from build123d import *

# Parameters (mm, degrees)
SKETCH1_R           = 19.05
BOSS_EXTRUDE1_DEPTH = 3.175
SKETCH2_R           = 12.065
CUT_EXTRUDE1_DEPTH  = 28.127211891
SKETCH3_R           = 13.335
CUT_EXTRUDE2_DEPTH  = 1.5875
BOSS_EXTRUDE2_START = 15.24
SKETCH4_W           = 6.35
SKETCH4_H           = 6.35
BOSS_EXTRUDE2_DEPTH = 9.525
FILLET1_R           = 2.54
SKETCH5_R           = 1.7272
CUT_EXTRUDE3_DEPTH  = 7.62
FILLET2_R           = 1.3208
FILLET3_R           = 0.127
SKETCH6_R           = 1.1303
CUT_EXTRUDE4_DEPTH  = 32.405228218


with BuildPart() as part:
    # Sketch1 → Boss-Extrude1 (new body)
    with BuildSketch(Plane.XY):
        Circle(SKETCH1_R)
    extrude(amount=BOSS_EXTRUDE1_DEPTH)

    # Sketch2 → Cut-Extrude1 (cut, through all)
    with BuildSketch(Plane.XY.offset(3.175)):
        Circle(SKETCH2_R)
    extrude(amount=-CUT_EXTRUDE1_DEPTH, mode=Mode.SUBTRACT)

    # Sketch3 → Cut-Extrude2 (cut)
    with BuildSketch(Plane.XY.offset(3.175)):
        Circle(SKETCH3_R)
    extrude(amount=-CUT_EXTRUDE2_DEPTH, mode=Mode.SUBTRACT)

    # Sketch4 → Boss-Extrude2 (add)
    with BuildSketch(Plane(origin=(0, 0, 0), x_dir=(0, 0, -1), z_dir=(1, 0, 0)).offset(BOSS_EXTRUDE2_START)):
        with Locations((-3.175, 0)):
            Rectangle(SKETCH4_W, SKETCH4_H)
    extrude(amount=BOSS_EXTRUDE2_DEPTH)

    # Fillet1
    fillet1_edges = [part.edges().sort_by_distance(p)[0] for p in [
        (18.783553311, -3.175, 1.5875),
        (18.783553311, 3.175, 1.5875),
    ]]
    fillet(fillet1_edges, radius=FILLET1_R)

    # Sketch5 → Cut-Extrude3 (cut)
    with BuildSketch(Plane(origin=(24.765, 0, 0), x_dir=(0, 0, -1), z_dir=(1, 0, 0))):
        with Locations((-3.175, 0)):
            Circle(SKETCH5_R)
    extrude(amount=-CUT_EXTRUDE3_DEPTH, mode=Mode.SUBTRACT)

    # Fillet2
    fillet2_edges = [part.edges().sort_by_distance(p)[0] for p in [
        (15.24, 0, 3.175),
        (15.24, 0, 6.35),
    ]]
    fillet(fillet2_edges, radius=FILLET2_R)

    # Fillet3
    # the kernel refuses this fillet: 0.127 mm, written as the material it takes off along each edge
    with BuildSketch(Plane(origin=(0, 0, 3.175), x_dir=(1, 0, 0), z_dir=(0, -1, 0))) as fillet3_piece_1:
        with BuildLine():
            CenterArc((13.335 + FILLET3_R, -FILLET3_R), FILLET3_R, 90, 90)
            Line((13.335, -FILLET3_R), (13.335, 0))
            Line((13.335, 0), (13.335 + FILLET3_R, 0))
        make_face()
    revolve(axis=Axis((0, 0, 3.175), (0, 0, 1)), mode=Mode.SUBTRACT)
    with BuildSketch(Plane(origin=(0, 0, 1.5875), x_dir=(1, 0, 0), z_dir=(0, -1, 0))) as fillet3_piece_2:
        with BuildLine():
            CenterArc((12.065 + FILLET3_R, -FILLET3_R), FILLET3_R, 90, 90)
            Line((12.065, -FILLET3_R), (12.065, 0))
            Line((12.065, 0), (12.065 + FILLET3_R, 0))
        make_face()
    revolve(axis=Axis((0, 0, 1.5875), (0, 0, 1)), mode=Mode.SUBTRACT)
    with BuildSketch(Plane(origin=(16.5608, -3.175, 6.35), x_dir=(0, 0, -1), z_dir=(1, 0, 0))) as fillet3_piece_3:
        with BuildLine():
            CenterArc((FILLET3_R, FILLET3_R), FILLET3_R, 180, 90)
            Line((0, FILLET3_R), (0, 0))
            Line((0, 0), (FILLET3_R, 0))
        make_face()
    extrude(amount=8.5217, mode=Mode.SUBTRACT)
    with BuildSketch(Plane(origin=(16.5608, 3.175, 6.35), x_dir=(0, 0, -1), z_dir=(1, 0, 0))) as fillet3_piece_4:
        with BuildLine():
            CenterArc((FILLET3_R, -FILLET3_R), FILLET3_R, 90, 90)
            Line((0, -FILLET3_R), (0, 0))
            Line((0, 0), (FILLET3_R, 0))
        make_face()
    extrude(amount=8.5217, mode=Mode.SUBTRACT)
    with BuildSketch(Plane(origin=(0, 0, 3.175), x_dir=(0.9643291947502942, 0.2647058823529412, 0), z_dir=(0.2647058823529412, -0.9643291947502942, 0))) as fillet3_piece_5:
        with BuildLine():
            CenterArc((19.05 - FILLET3_R, -FILLET3_R), FILLET3_R, 0, 90)
            Line((19.05 - FILLET3_R, 0), (19.05, 0))
            Line((19.05, 0), (19.05, -FILLET3_R))
        make_face()
    revolve(axis=Axis((0, 0, 3.175), (0, 0, 1)), revolution_arc=329.301045966, mode=Mode.SUBTRACT)
    with BuildSketch(Plane(origin=(20.819867315, 5.715, 3.175), x_dir=(0.12470900704731759, -0.9921933599663284, 0), z_dir=(0.9921933599663284, 0.12470900704731759, 0))) as fillet3_piece_6_section:
        with BuildLine():
            CenterArc((2.54 + FILLET3_R, FILLET3_R), FILLET3_R, 180, 90)
            Line((2.54, FILLET3_R), (2.54, 0))
            Line((2.54, 0), (2.54 + FILLET3_R, 0))
        make_face()
    fillet3_piece_6 = revolve(axis=Axis((20.819867315, 5.715, 3.175), (0, 0, -1)), revolution_arc=81.814474605, mode=Mode.PRIVATE)
    fillet3_piece_6 = split(fillet3_piece_6, bisect_by=Plane(origin=(19.258112291, 3.175, 3.13928763), z_dir=(0, 1, 0)), keep=Keep.TOP, mode=Mode.PRIVATE)
    add(fillet3_piece_6, mode=Mode.SUBTRACT)
    with BuildSketch(Plane(origin=(20.819867315, -5.715, 3.175), x_dir=(0.12470900704731899, 0.9921933599663282, 0), z_dir=(0.9921933599663282, -0.12470900704731899, 0))) as fillet3_piece_7_section:
        with BuildLine():
            CenterArc((2.54 + FILLET3_R, -FILLET3_R), FILLET3_R, 90, 90)
            Line((2.54 + FILLET3_R, 0), (2.54, 0))
            Line((2.54, 0), (2.54, -FILLET3_R))
        make_face()
    fillet3_piece_7 = revolve(axis=Axis((20.819867315, -5.715, 3.175), (0, 0, 1)), revolution_arc=81.814474605, mode=Mode.PRIVATE)
    fillet3_piece_7 = split(fillet3_piece_7, bisect_by=Plane(origin=(19.258112291, -3.175, 3.13928763), z_dir=(0, -1, 0)), keep=Keep.TOP, mode=Mode.PRIVATE)
    add(fillet3_piece_7, mode=Mode.SUBTRACT)
    with BuildSketch(Plane(origin=(15.24, -3.175, 4.4958), x_dir=(1, 0, 0), z_dir=(0, 0, 1)), Plane(origin=(15.24, 3.175, 5.0292), x_dir=(1, 0, 0), z_dir=(0, 0, -1))) as fillet3_piece_8:
        with BuildLine():
            CenterArc((FILLET3_R, FILLET3_R), FILLET3_R, 180, 90)
            Line((0, FILLET3_R), (0, 0))
            Line((0, 0), (FILLET3_R, 0))
        make_face()
    extrude(amount=0.5334, mode=Mode.SUBTRACT)
    with BuildSketch(Plane(origin=(16.5608, -3.175, 5.0292), x_dir=(-1, 0, 0), z_dir=(0, 0, -1))) as fillet3_piece_9:
        with BuildLine():
            CenterArc((1.3208 - FILLET3_R, FILLET3_R), FILLET3_R, 270, 90)
            Line((1.3208, FILLET3_R), (1.3208, 0))
            Line((1.3208, 0), (1.3208 - FILLET3_R, 0))
        make_face()
    revolve(axis=Axis((16.5608, -3.175, 5.0292), (0, 1, 0)), revolution_arc=90, mode=Mode.SUBTRACT)
    with BuildSketch(Plane(origin=(16.5608, 3.175, 5.0292), x_dir=(-1, 0, 0), z_dir=(0, 0, -1))) as fillet3_piece_10:
        with BuildLine():
            CenterArc((1.3208 - FILLET3_R, -FILLET3_R), FILLET3_R, 0, 90)
            Line((1.3208, -FILLET3_R), (1.3208, 0))
            Line((1.3208, 0), (1.3208 - FILLET3_R, 0))
        make_face()
    revolve(axis=Axis((16.5608, 3.175, 5.0292), (0, 1, 0)), revolution_arc=90, mode=Mode.SUBTRACT)
    with BuildSketch(Plane(origin=(13.9192, 3.175, 4.4958), x_dir=(-0.23816998714710041, 0, -0.9712234846946144), z_dir=(-0.9712234846946144, 0, 0.23816998714710041))) as fillet3_piece_11_section:
        with BuildLine():
            CenterArc((1.3208 + FILLET3_R, FILLET3_R), FILLET3_R, 180, 90)
            Line((1.3208, FILLET3_R), (1.3208, 0))
            Line((1.3208, 0), (1.3208 + FILLET3_R, 0))
        make_face()
    fillet3_piece_11 = revolve(axis=Axis((13.9192, 3.175, 4.4958), (0, -1, 0)), revolution_arc=103.778556657, mode=Mode.PRIVATE)
    fillet3_piece_11 = split(fillet3_piece_11, bisect_by=Plane(origin=(14.878561501, 3.139057971, 3.175), z_dir=(0, 0, 1)), keep=Keep.TOP, mode=Mode.PRIVATE)
    add(fillet3_piece_11, mode=Mode.SUBTRACT)
    with BuildSketch(Plane(origin=(13.9192, -3.175, 4.4958), x_dir=(-0.23816998714710186, 0, -0.9712234846946141), z_dir=(-0.9712234846946141, 0, 0.23816998714710186))) as fillet3_piece_12_section:
        with BuildLine():
            CenterArc((1.3208 + FILLET3_R, -FILLET3_R), FILLET3_R, 90, 90)
            Line((1.3208 + FILLET3_R, 0), (1.3208, 0))
            Line((1.3208, 0), (1.3208, -FILLET3_R))
        make_face()
    fillet3_piece_12 = revolve(axis=Axis((13.9192, -3.175, 4.4958), (0, -1, 0)), revolution_arc=103.778556657, mode=Mode.PRIVATE)
    fillet3_piece_12 = split(fillet3_piece_12, bisect_by=Plane(origin=(14.878561477, -3.139057971, 3.175), z_dir=(0, 0, 1)), keep=Keep.TOP, mode=Mode.PRIVATE)
    add(fillet3_piece_12, mode=Mode.SUBTRACT)

    # Sketch6 → Cut-Extrude4 (cut, through all)
    with BuildSketch(Plane.XY.offset(3.175)):
        with Locations((-16.66875, 0)):
            Circle(SKETCH6_R)
        with Locations((0, 16.66875)):
            Circle(SKETCH6_R)
        with Locations((0, -16.66875)):
            Circle(SKETCH6_R)
    extrude(amount=-CUT_EXTRUDE4_DEPTH, mode=Mode.SUBTRACT)


solid = part.part
Source: CAD feature listing. Evaluate the final solid. Frame: model axes, mm. A direction names the side the tool comes from. Coordinates: 2 decimals unless noted, no trailing zeros. Loops run counter-clockwise (first coordinate to the right, second up) from the corner with the lowest first, then second, coordinate; pieces in that order, holes last. Notation, with made-up numbers: M -26,-7 L 0,-7 A24 ccw 0,12 Z; hole C 73,11 d7. An arc over 180 degrees is marked long. Answer in a Markdown table with one row per item.
Q1. Set-up query: faces 4 (the cylindrical face through (11.51, 3.62, 0.74)), 5 (the cylindrical face through (-1.74, 13.22, 2.33)), 6 (the cylindrical face through (21.008, 1.167, 4.448)). Return all of +Z, -Z, +X, -X, +Y, -Y with unobstructed straight access to the full face (end or side cutting, diameter ignored); none if empty.
Answers below:
| item | result |
|---|---|
| face 4 | +Z, -Z |
| face 5 | +Z |
| face 6 | +X |
Q2. Section A-A on x = 0. State how many separate pieces and enclosed holes the cut face has, plus the area to 3 significant figures.
Answers below:
| item | result |
|---|---|
| separate pieces | 4 |
| enclosed holes | 0 |
| area | 25.9 mm^2 |
Q3. First-contact query: pin 1 (1.9 mm diameter, centred on x = 21, z = 3.5, fed in from -Y); pin 2 (10 mm diameter, centred on x = -13.5, y = 8.5, fed in from +Z) (3 decimals); pin 3 (3 mm diameter, centred on x = 3.5, z = 2.5, fed in from +Y); pin 4 (1.8 mm diameter, centred on x = 0, y = 16.67, fed in from -Z). Flat tips, straight axial feed; report the tip coordinate or a pass-through.
Answers below:
| item | result |
|---|---|
| pin 1 | stops at y = -3.26 |
| pin 2 | stops at z = 3.175 |
| pin 3 | stops at y = 18.94 |
| pin 4 | passes through |
Q4. Ray query, probe 1 along Y at (x, z) = (0, 0.9) (3 decimals); probe 2 along Y at (x, z) = (0, 2.3) (3 decimals); probe 3 along X at (y, z) = (1, 3) (3 decimals). Return the intervals inside material, ascending. Write a range as from..to.
Answers below:
| item | result |
|---|---|
| probe 1 | y = -19.05..-17.799, -15.538..-12.065, 12.065..15.538, 17.799..19.05 |
| probe 2 | y = -19.05..-17.799, -15.538..-13.335, 13.335..15.538, 17.799..19.05 |
| probe 3 | x = -19.024..-17.196, -16.142..-13.297, 13.297..17.145 |
Q5. Draft query along Y for faces 1 (the cylindrical face through (-0.15, -15.55, 1.61)), 2 (the flat face through (21, -3.175, 4)), 3 (the flat face through (21, 3.175, 4)). Return one class per face: pulls with the +Y half, pulls with the -Y half, needs draft (parallel to the pull), parting line crosses it, or undercut.
Answers below:
| item | result |
|---|---|
| face 1 | undercut |
| face 2 | pulls with the -Y half |
| face 3 | pulls with the +Y half |
Q6. Section C-C on z = 0.5. Return the cut outline in (x, y) (3 decimals).
Answers below:
| item | result |
|---|---|
| outline | M 18.37,-5.043 A2.54 cw 20.82,-3.175 L 24.765,-3.175 L 24.765,3.175 L 20.82,3.175 A2.54 cw 18.37,5.043 A19.05 ccw long Z; hole C -16.669,0 d2.261; hole C 0,0 d24.13; hole C 0,-16.669 d2.261; hole C 0,16.669 d2.261 |
